Autodesk Inventor part; units mm, degrees
ref_plane "YZ Plane" through (0, 0, 0) normal (1, 0, 0) x (0, 1, 0)
ref_plane "XZ Plane" through (0, 0, 0) normal (0, 1, 0) x (-1, 0, 0)
ref_plane "XY Plane" through (0, 0, 0) normal (0, 0, 1) x (1, 0, 0)
sketch "Sketch1" plane through (0, 0, 0) normal (1, 0, 0) x (0, 1, 0)
  line L0 (-4.1396, 10.001) -> (4.1446, 9.999)
  line L1 (4.1446, 9.999) -> (10.001, 4.1396)
  line L2 (10.001, 4.1396) -> (9.999, -4.1446)
  line L3 (9.999, -4.1446) -> (4.1396, -10.001)
  line L4 (4.1396, -10.001) -> (-4.1446, -9.999)
  line L5 (-4.1446, -9.999) -> (-10.001, -4.1396)
  line L6 (-10.001, -4.1396) -> (-9.999, 4.1446)
  line L7 (-9.999, 4.1446) -> (-4.1396, 10.001)
  circle A0 centre (0, 0) radius 3
  dimension "d0" = 10
  dimension "d1" = 6
extrude "Extrusion1" add sketch "Sketch1" along normal blind 3
properties part number "Nuy"
The listing builds one solid part. Answer for the finished solid, in the listing's coordinates (mm). Coordinates: 2 decimals unless noted, no trailing zeros. Write each loop counter-clockwise with the first axis right and the second up, starting at its lowest first coordinate (ties: lowest second). Pieces come first, ordered by that corner, then holes.
Q1. Section C-C, the plane x = 0.6 is taken. Write down the section's boundary in (y, z).
Returned:
outline: (-10, -4.14) - (-4.14, -10) - (4.14, -10) - (10, -4.14) - (10, 4.14) - (4.14, 10) - (-4.14, 10) - (-10, 4.14) - close; hole circle Ø6 at (0, 0)
Q2. Section D-D, the plane y = -7.25 is taken. Write down the section's boundary in (x, z).
Returned:
outline: (0, -6.89) - (3, -6.89) - (3, 6.89) - (0, 6.89) - close
Q3. Given P1, Ø1.5, axis at x = 1, z = 6.5, coming from the -Y side, flat-ended and moving along its own axis, determine where the tip first touches the part or whether it passes through.
Returned:
P1: stops at y = -8.39
Q4. Section A-A, the plane y = 0 is taken. Write down the section's boundary in (x, z).
Returned:
outline: (0, -10) - (3, -10) - (3, -3) - (0, -3) - close; (0, 3) - (3, 3) - (3, 10) - (0, 10) - close
Q5. Find the intervals of material crossed by line 1 along Z through (x, y) = (2.2, 0); line 2 along Z through (x, y) = (0.8, -0.75); line 3 along Y through (x, z) = (2.45, -3.5), in increasing order.
Returned:
line 1: z = -10 to -3, 3 to 10
line 2: z = -10 to -2.9, 2.9 to 10
line 3: y = -10 to 10
